```python
from build123d import *

# Parameters (mm, degrees)
F0_R     = 3
F1_DEPTH = 340
F2_W     = 40
F2_H     = 20
F3_DEPTH = 40
F4_R     = 15
F5_DEPTH = 10


with BuildPart() as f1:
    # F0 (on Front) → F1 (new body)
    with BuildSketch(Plane.XZ):
        Circle(F0_R)
    extrude(amount=F1_DEPTH)

    # F2 (on Front) → F3 (join)
    with BuildSketch(Plane.XZ):
        Rectangle(F2_W, F2_H)
    extrude(amount=F3_DEPTH)

    # F4 (on face) → F5 (cut)
    with BuildSketch(Plane.XY.offset(10)):
        with Locations((0, -20)):
            Circle(F4_R)
    extrude(amount=-F5_DEPTH, mode=Mode.SUBTRACT)


solid = f1.part
```
Source: CAD feature listing. Evaluate the final solid. Frame: model axes, mm. A direction names the side the tool comes from. Round coordinates to 2 decimals unless told otherwise and drop trailing zeros. Loops run counter-clockwise (first coordinate to the right, second up) from the corner with the lowest first, then second, coordinate; pieces in that order, holes last.
1. Section query C-C on z = -6.5. Output: boundary loops of the cut face in (x, y), and give its area (3 significant figures).
2. Section query A-A on y = -20. Output: boundary loops of the cut face in (x, z).
3. Contact query for flat-ended pins moving along their axis: pin 1 (10 mm diameter, centred on x = -7, z = 5, fed in from -Y); pin 2 (8 mm diameter, centred on x = 1, y = -276.5, fed in from -Z); pin 3 (1 mm diameter, centred on x = -8.5, z = -5, fed in from +Y). Output: stop coordinate, or through.
4. Section query B-B on x = 0. Output: boundary loops of the cut face in (y, z), and give its area (3 significant figures).
5. Section query D-D on y = -161.5. Output: boundary loops of the cut face in (x, z), and give its area (3 significant figures).
6. Access query for faces 5 (the flat face through (-20, -20, 0)), 6 (the cylindrical face through (-3, -188, 0)). Directions: +Z, -Z, +X, -X, +Y, -Y. A direction counts if a zero-diameter tool reaches every point of the face in a straight line with its end or side. Return the directions, or none.
7. Ray query, L1, parallel to Y at x = 0, z = 5.25; L2, parallel to Y at x = 0, z = 2.75; L3, parallel to Y at x = 16, z = 4. Return the intervals inside material, ascending.
8. Mould query, pull axis Y, two halves, no side actions, for faces 1 (the flat face through (0, -20, 0)), 2 (the flat face through (20, -20, 0)), 3 (the flat face through (0, -40, 5)), 4 (the cylindrical face through (-3.252, -34.643, 5.07)). Classes: released by +Y, released by -Y, zero draft, split by the parting line, or undercut.
Answers below:
1. outline: (-20, -40) - (20, -40) - (20, 0) - (-20, 0) - close
1. area: 1,600 mm2
2. outline: (-20, -10) - (20, -10) - (20, 10) - (15, 10) - (15, 0) - (-15, 0) - (-15, 10) - (-20, 10) - close
3. pin 1: stops at y = -40
3. pin 2: stops at z = -3
3. pin 3: stops at y = 0
4. outline: (-340, -3) - (-40, -3) - (-40, -10) - (0, -10) - (0, 10) - (-5, 10) - (-5, 0) - (-35, 0) - (-35, 10) - (-40, 10) - (-40, 3) - (-340, 3) - close
4. area: 2,300 mm2
5. outline: circle Ø6 at (0, 0)
5. area: 28.3 mm2
6. face 5: +Z, -Z, -X, +Y, -Y
6. face 6: -Y
7. L1: y = -40 to -35, -5 to 0
7. L2: y = -340 to -35, -5 to 0
7. L3: y = -40 to 0
8. face 1: undercut
8. face 2: zero draft
8. face 3: released by -Y
8. face 4: undercut
